Design review of the part built by this model. Coordinates are the model's own, in mm. A direction names the side the tool comes from. Coordinates: 2 decimals unless noted, no trailing zeros. Write each loop counter-clockwise with the first axis right and the second up, starting at its lowest first coordinate (ties: lowest second). Pieces come first, ordered by that corner, then holes.
Q1. Take a section at A-A (y = -1.25). Give the boundary of the cut face in (x, z).
Q2. Take a section at D-D (x = -6.5). Give the boundary of the cut face in (y, z), and give its area (4 significant figures).
Q3. For probe 1 along X at (y, z) = (1.5, -14); probe 2 along X at (y, z) = (2.65, -13.78); probe 3 along X at (y, z) = (-3, -14), list the stretches that pass through material, from the lowest coordinate up.
Q4. Machinability: for faces 5 (the cylindrical face through (-41.07, -2.46, -14.24)), 6 (the flat face through (-18, 2, -11.28)), 7 (the cylindrical face through (-34.13, 2.51, -14.24)), which of the approach directions +Z, -Z, +X, -X, +Y, -Y give a long, thin tool a straight path to every point of the face, cutting with its end or side? Answer none if there is none.
Q5. Insertion check: pin 1 (4.5 mm diameter, centred on x = 47, z = -24.5, fed in from -Y); pin 2 (1.5 mm diameter, centred on x = -48, y = -1, fed in from -Z); pin 3 (3 mm diameter, centred on x = -39, y = -2, fed in from -Z); pin 4 (3 mm diameter, centred on x = 23.5, y = -4, fed in from +Z). Each pin has a flat end and moves straight along its axis. Give the tip position at first contact, or say it passes through.
Q6. Mouldability with a two-part tool opening along X and no side actions: class faces 1 (the cylindrical face through (20.39, -1.45, -14.32)), 2 (the cylindrical face through (54.95, 1.52, -29.68)), 3 (the flat face through (-48, -1, -23.25)), 4 (the flat face through (-55.55, 1, 0)) as pulls with the +X half, pulls with the -X half, needs draft (parallel to the pull), parting line crosses it, or undercut.
Q7. Take a section at B-B (x = -37.6). Give the boundary of the cut face in (y, z).
Q8. Take a section at C-C (z = -13.78). State how many separate pieces and enclosed holes the cut face has, and give its area (3 significant figures).
```python
from build123d import *

# Parameters (mm, degrees)
SKETCH1_W           = 111.1
SKETCH1_H           = 60.5
BOSS_EXTRUDE1_DEPTH = 3
SKETCH9_W           = 5
SKETCH9_H           = 4
BOSS_EXTRUDE5_DEPTH = 3
FILLET1_R           = 2
SKETCH10_R          = 2.5
SKETCH10_W          = 4.2
SKETCH10_H          = 8.55
CUT_EXTRUDE1_DEPTH  = 10
SKETCH11_R          = 3.5
CUT_EXTRUDE2_DEPTH  = 1
SKETCH12_R          = 3.5
SKETCH12_R_2        = 2.5
BOSS_EXTRUDE6_DEPTH = 5


with BuildPart() as part:
    # Sketch1 → Boss-Extrude1 (new body)
    with BuildSketch(Plane(origin=(0, 0, 0), x_dir=(1, 0, 0), z_dir=(0, 1, 0))):
        Rectangle(SKETCH1_W, SKETCH1_H)
    extrude(amount=BOSS_EXTRUDE1_DEPTH)

    # Sketch9 → Boss-Extrude5 (add)
    with BuildSketch(Plane.XZ):
        with Locations((-48.05, -25.25)):
            Rectangle(SKETCH9_W, SKETCH9_H)
        with Locations((48.05, -25.25)):
            Rectangle(SKETCH9_W, SKETCH9_H)
    extrude(amount=BOSS_EXTRUDE5_DEPTH)

    # Fillet1
    fillet1_edges = [part.edges().sort_by_distance(p)[0] for p in [
        (-55.55, 1.5, -30.25),
        (55.55, 1.5, -30.25),
        (55.55, 1.5, 30.25),
        (-55.55, 1.5, 30.25),
    ]]
    fillet(fillet1_edges, radius=FILLET1_R)

    # Sketch10 → Cut-Extrude1 (cut)
    with BuildSketch(Plane(origin=(0, 3, 0), x_dir=(1, 0, 0), z_dir=(0, 1, 0))):
        with Locations(Location((-37.6, 13.78, 0), (0, 0, 270))):
            Circle(SKETCH10_R)
        with Locations(Location((17.95, 13.78, 0), (0, 0, 270))):
            Circle(SKETCH10_R)
        with Locations((37.55, 15.555)):
            Rectangle(SKETCH10_W, SKETCH10_H)
        with Locations((-18, 15.555)):
            Rectangle(SKETCH10_W, SKETCH10_H)
    extrude(amount=-CUT_EXTRUDE1_DEPTH, mode=Mode.SUBTRACT)

    # Sketch11 → Cut-Extrude2 (cut)
    with BuildSketch(Plane(origin=(0, 3, 0), x_dir=(1, 0, 0), z_dir=(0, 1, 0))):
        with Locations(Location((-37.6, 13.78, 0), (0, 0, 270))):
            Circle(SKETCH11_R)
        with Locations(Location((17.95, 13.78, 0), (0, 0, 270))):
            Circle(SKETCH11_R)
    extrude(amount=-CUT_EXTRUDE2_DEPTH, mode=Mode.SUBTRACT)

    # Sketch12 → Boss-Extrude6 (add)
    # profile 1 of 2: a face of its own
    with BuildSketch(Plane.XZ):
        with Locations(Location((17.95, -13.78, 0), (0, 0, 90))):
            Circle(SKETCH12_R)
        with Locations(Location((17.95, -13.78, 0), (0, 0, 90))):
            Circle(SKETCH12_R_2, mode=Mode.SUBTRACT)
    # profile 2 of 2: a face of its own
    with BuildSketch(Plane.XZ):
        with Locations(Location((-37.6, -13.78, 0), (0, 0, 90))):
            Circle(SKETCH12_R)
        with Locations(Location((-37.6, -13.78, 0), (0, 0, 90))):
            Circle(SKETCH12_R_2, mode=Mode.SUBTRACT)
    extrude(amount=BOSS_EXTRUDE6_DEPTH)


solid = part.part
```
Response:
1. outline: (-50.55, -27.25) - (-45.55, -27.25) - (-45.55, -23.25) - (-50.55, -23.25) - close; circle Ø7 at (-37.6, -13.78); circle Ø7 at (17.95, -13.78); (45.55, -27.25) - (50.55, -27.25) - (50.55, -23.25) - (45.55, -23.25) - close; hole circle Ø5 at (-37.6, -13.78); hole circle Ø5 at (17.95, -13.78)
2. outline: (0, -30.25) - (3, -30.25) - (3, 30.25) - (0, 30.25) - close
2. area: 181.5 mm2
3. probe 1: x = -55.55 to -40.09, -35.11 to -20.1, -15.9 to 15.46, 20.44 to 35.45, 39.65 to 55.55
3. probe 2: x = -55.55 to -41.1, -34.1 to -20.1, -15.9 to 14.45, 21.45 to 35.45, 39.65 to 55.55
3. probe 3: x = -41.09 to -40.09, -35.11 to -34.11, 14.46 to 15.46, 20.44 to 21.44
4. face 5: -Y
4. face 6: +Y, -Y
4. face 7: +Y
5. pin 1: stops at y = -3
5. pin 2: stops at z = -27.25
5. pin 3: stops at z = -17.28
5. pin 4: passes through
6. face 1: undercut
6. face 2: pulls with the +X half
6. face 3: needs draft
6. face 4: pulls with the -X half
7. outline: (-5, -17.28) - (0, -17.28) - (0, -30.25) - (3, -30.25) - (3, -17.28) - (2, -17.28) - (2, -16.28) - (-5, -16.28) - close; (-5, -11.28) - (2, -11.28) - (2, -10.28) - (3, -10.28) - (3, 30.25) - (0, 30.25) - (0, -10.28) - (-5, -10.28) - close
8. separate pieces: 5
8. enclosed holes: 0
8. area: 294 mm2
